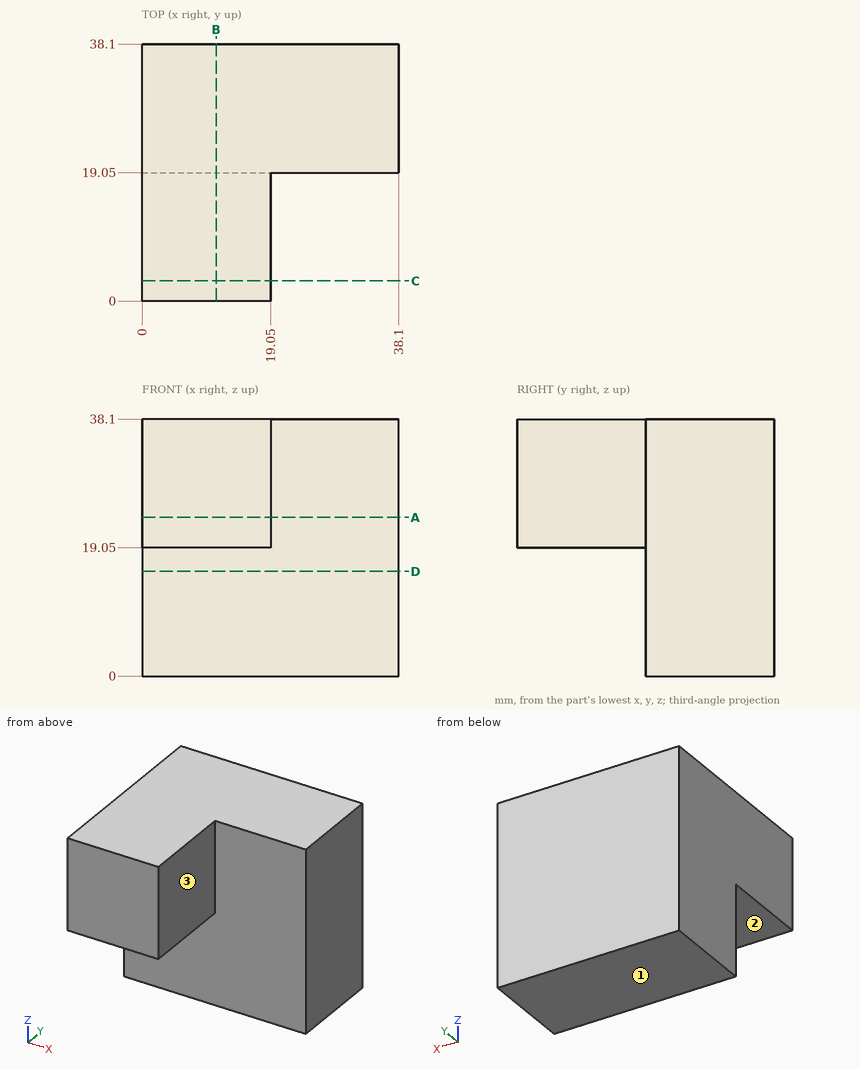
Design review of the part shown in the three views and the two pictorial views. Dimensions are in mm from the part's minimum x, y and z. A direction names the side the tool comes from. Give positions to 0.01 mm unless a question says otherwise; leave off trailing zeros. Write each loop counter-clockwise with the first axis right and the second up, starting at its lowest first coordinate (ties: lowest second). Pieces come first, ordered by that corner, then holes. Notation, with made-up numbers: (85, -28) - (93, -28) arc R24 cw to (93, 2) - close; hole circle Ø8 at (-26, 17.5). An arc over 180 degrees is marked (long way). Return JSON: item names as keys, results as strings. Group by question number.
(1) We need section C-C, the plane y = 3. Give the boundary of the cut face in (x, z), then the cut area to 3 significant figures.
(2) We need section B-B, the plane x = 11. Give the boundary of the cut face in (y, z).
(3) We need section A-A, the plane z = 23.5. Give the boundary of the cut face in (x, y), then the cut area to 3 significant figures.
(4) We need section D-D, the plane z = 15.5. Give the boundary of the cut face in (x, y), then the cut area to 3 significant figures.
(5) Machinability: for the marked faces 1, 2 and 3, which of the approach directions +Z, -Z, +X, -X, +Y, -Y give a long, thin tool a straight path to every point of the face, cutting with its end or side? Answer none if there is none.
(6) Insertion check: pin 1 (6 mm diameter, centred on y = 18, z = 19, fed in from -X); pin 2 (6 mm diameter, centred on x = 6, y = 4.5, fed in from -Z); pin 3 (8 mm diameter, centred on y = 14, z = 12, fed in from -X); pin 4 (11.5 mm diameter, centred on x = 26.5, z = 22.5, fed in from -Y). Each pin has a flat end and moves straight along its axis. Give the tip position at first contact, or say it passes through.
(7) To check wall thickness, follow probe 1 along Y at (x, z) = (26, 20); probe 2 along X at (y, z) = (17, 23). State the ranges of each line that lie inside material, in increasing order.
Reported:
{
 "1": {"outline": "(0, 19.05) - (19.05, 19.05) - (19.05, 38.1) - (0, 38.1) - close", "area": "363 mm2"},
 "2": {"outline": "(0, 19.05) - (19.05, 19.05) - (19.05, 0) - (38.1, 0) - (38.1, 38.1) - (0, 38.1) - close"},
 "3": {"outline": "(0, 0) - (19.05, 0) - (19.05, 19.05) - (38.1, 19.05) - (38.1, 38.1) - (0, 38.1) - close", "area": "1,090 mm2"},
 "4": {"outline": "(0, 19.05) - (38.1, 19.05) - (38.1, 38.1) - (0, 38.1) - close", "area": "726 mm2"},
 "5": {"face 1": "-Z, +X, -X, +Y, -Y", "face 2": "-Z, +X, -X, -Y", "face 3": "+Z, -Z, +X, -Y"},
 "6": {"pin 1": "stops at x = 0", "pin 2": "stops at z = 19.05", "pin 3": "passes through", "pin 4": "stops at y = 19.05"},
 "7": {"probe 1": "y = 19.05 to 38.1", "probe 2": "x = 0 to 19.05"}
}
